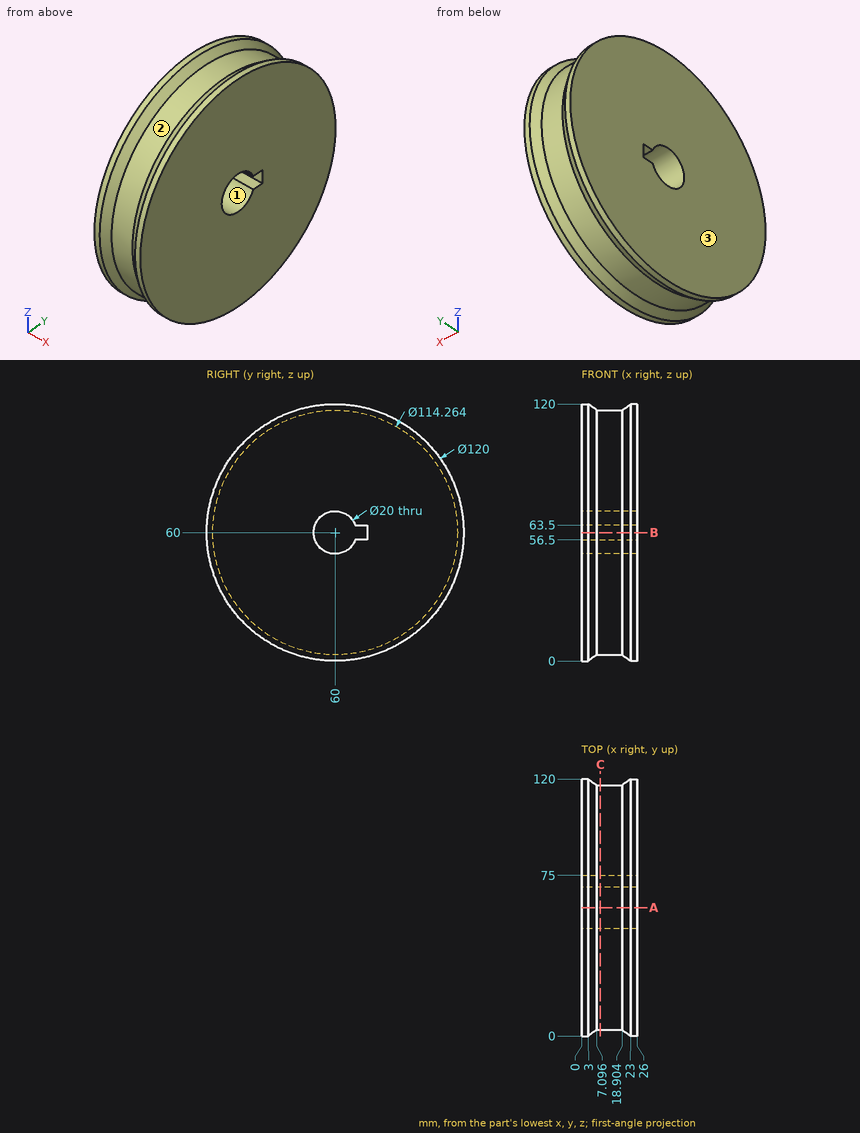
Can you work these out from the drawing? Everything is in mm from the part's minimum corner. Round coordinates to 2 decimals unless told otherwise and drop trailing zeros. Order: outer loops, then holes, each group sorted by start corner. A loop starts at its lowest first (then second) coordinate and runs counter-clockwise, first axis right, second up.
(1) I'm going to push flat-ended pins straight in: pin 1 (12 mm diameter, centred on x = 22, y = 92, fed in from +Z); pin 2 (2 mm diameter, centred on x = 12.5, z = 59, fed in from -Y); pin 3 (3 mm diameter, centred on x = 9.5, y = 72.5, fed in from +Z); pin 4 (12 mm diameter, centred on y = 60, z = 60, fed in from +X). Where does each tip first touch, or does it pass through?
Results are:
pin 1: stops at z = 114.03
pin 2: stops at y = 2.87
pin 3: stops at z = 116.06
pin 4: passes through
(2) If we section it at C-C (x = 8.75): Please give me the cut outline in (y, z), plus the area to 3 significant figures.
Results are:
outline: circle Ø114.26 at (60, 60); hole (69.37, 56.5) - (75, 56.5) - (75, 63.5) - (69.37, 63.5) arc R10 ccw (long way) to start
area: 9,900 mm2
(3) If we section it at A-A (y = 60): Please give me the cut outline in (x, z).
Results are:
outline: (0, 0) - (3, 0) - (7.1, 2.87) - (18.9, 2.87) - (23, 0) - (26, 0) - (26, 50) - (0, 50) - close; (0, 70) - (26, 70) - (26, 120) - (23, 120) - (18.9, 117.13) - (7.1, 117.13) - (3, 120) - (0, 120) - close
(4) If we section it at B-B (z = 60): Please give me the cut outline in (x, y).
Results are:
outline: (0, 0) - (3, 0) - (7.1, 2.87) - (18.9, 2.87) - (23, 0) - (26, 0) - (26, 50) - (0, 50) - close; (0, 75) - (26, 75) - (26, 120) - (23, 120) - (18.9, 117.13) - (7.1, 117.13) - (3, 120) - (0, 120) - close
(5) We'd pull the mould along X, two halves only. Please class the marked faces 1, 2 and 3: +X half, -X half, draft (parallel to the pull), parting line (faces both ways), or undercut.
Results are:
face 1: draft
face 2: undercut
face 3: -X half
(6) If I drill on L1, parallel to Y at x = 18.5, z = 60; L2, parallel to Z at x = 12.75, y = 60; L3, parallel to Z at x = 1.75, y = 59.5, over which ranges is the centre line in solid material (lowest first)?
Results are:
L1: y = 2.87 to 50, 75 to 117.13
L2: z = 2.87 to 50, 70 to 117.13
L3: z = 0 to 50.01, 69.99 to 120
